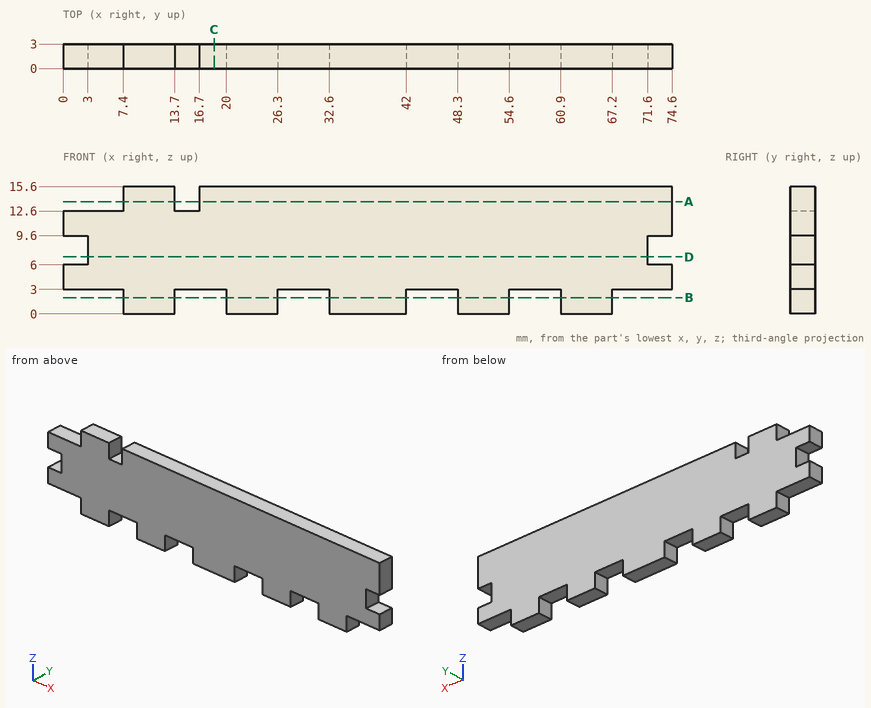
Check sheet for the drawn part. Datum: minimum x, y, z corner. Units: mm. Give positions to 0.01 mm unless a question says otherwise; leave off trailing zeros. Write each loop counter-clockwise with the first axis right and the second up, starting at its lowest first coordinate (ties: lowest second). Pieces come first, ordered by that corner, then holes.
(1) Gauge pin test, flat ends, axial feed: pin 1 (0.9 mm diameter, centred on y = 1, z = 1.5, fed in from +X); pin 2 (1.5 mm diameter, centred on y = 1.5, z = 2, fed in from -X); pin 3 (1.5 mm diameter, centred on x = 2, y = 1.5, fed in from +Z). Record the tip position at first contact, or that the pin passes through.
(2) Material ranges on line 1 (X direction, y = 1.55, z = 13.75); line 2 (Z direction, x = 30.5, y = 1.7); line 3 (Z direction, x = 15.5, y = 1.6), recorded low to high.
(3) Cross-section at A-A (z = 13.75). Enter the section's corners in (x, y), plus the area to 3 significant figures.
(4) Cross-section at C-C (x = 18.5). Enter the section's corners in (y, z).
(5) Cross-section at D-D (z = 7). Enter the section's corners in (x, y).
(6) Cross-section at B-B (z = 2). Enter the section's corners in (x, y), plus the area to 3 significant figures.
Worked out:
1. pin 1: stops at x = 67.2
1. pin 2: stops at x = 7.4
1. pin 3: stops at z = 12.6
2. line 1: x = 7.4 to 13.7, 16.7 to 74.6
2. line 2: z = 3 to 15.6
2. line 3: z = 3 to 12.6
3. outline: (7.4, 0) - (13.7, 0) - (13.7, 3) - (7.4, 3) - close; (16.7, 0) - (74.6, 0) - (74.6, 3) - (16.7, 3) - close
3. area: 193 mm2
4. outline: (0, 3) - (3, 3) - (3, 15.6) - (0, 15.6) - close
5. outline: (3, 0) - (71.6, 0) - (71.6, 3) - (3, 3) - close
6. outline: (7.4, 0) - (13.7, 0) - (13.7, 3) - (7.4, 3) - close; (20, 0) - (26.3, 0) - (26.3, 3) - (20, 3) - close; (32.6, 0) - (42, 0) - (42, 3) - (32.6, 3) - close; (48.3, 0) - (54.6, 0) - (54.6, 3) - (48.3, 3) - close; (60.9, 0) - (67.2, 0) - (67.2, 3) - (60.9, 3) - close
6. area: 104 mm2
